```python
from build123d import *

# Parameters (mm, degrees)
SKETCH1_R           = 2.25
BOSS_EXTRUDE1_DEPTH = 3.5


with BuildPart() as part:
    # Sketch1 → Boss-Extrude1 (new body)
    with BuildSketch(Plane.XY):
        with BuildLine():
            Line((-100, 100), (-100, -100))
            Line((-100, -100), (-60.466933112, -100))
            ThreePointArc((-60.466933112, -100), (-38.490639688, 54.111358665), (92.5, -30))
            ThreePointArc((92.5, -30), (84.111358665, -68.490639688), (60.466933112, -100))
            Line((60.466933112, -100), (100, -100))
            Line((100, -100), (100, 32))
            Line((100, 32), (32, 100))
            Line((32, 100), (-100, 100))
        make_face()
        with Locations((-96.15, -96.15)):
            Circle(SKETCH1_R, mode=Mode.SUBTRACT)
        with Locations((96.15, -96.15)):
            Circle(SKETCH1_R, mode=Mode.SUBTRACT)
        with Locations((-96.15, 96.15)):
            Circle(SKETCH1_R, mode=Mode.SUBTRACT)
    extrude(amount=BOSS_EXTRUDE1_DEPTH)


solid = part.part
```
Design review of the part built by this model. Coordinates are the model's own, in mm. Coordinates: 2 decimals unless noted, no trailing zeros. Order: outer loops, then holes, each group sorted by start corner. A loop starts at its lowest first (then second) coordinate and runs counter-clockwise, first axis right, second up. Notation, with made-up numbers: M 4.25,67 L 31.25,67 A18 cw 31.25,71 Z; hole C 63.25,24.25 d9. An arc over 180 degrees is marked long. Answer as a JSON object with one key per item and string values. Group by question number.
1) Add section A-A, the plane y = 60. Write out the cut boundary in (x, z).
2) Mouldability with a two-part tool opening along X and no side actions: class faces 1 (the cylindrical face through (-94.07, -97.01, 1.73)), 2 (the flat face through (-38, 60, 3.5)), 3 (the flat face through (66, 66, 2)) as pulls with the +X half, pulls with the -X half, needs draft (parallel to the pull), parting line crosses it, or undercut.
3) Add section D-D, the plane x = 36. Write out the cut boundary in (y, z), then the cut area to 3 significant figures.
4) Add section B-B, the plane z = 2.85. Write out the cut boundary in (x, y), then the cut area to 3 significant figures.
5) Add section C-C, the plane x = -69. Write out the cut boundary in (y, z), then the cut area to 3 significant figures.
6) Wall thickness on L1, parallel to Y at x = -96.15, z = 2.6; L2, parallel to X at y = -14, z = 3.1; L3, parallel to Y at x = -69.5, z = 0.85: over which ranges is each line inside the solid? List them lowest first.
Computed values:
{
 "1": {"outline": "M -100,0 L -21.36,0 L -21.36,3.5 L -100,3.5 Z; M 21.36,0 L 72,0 L 72,3.5 L 21.36,3.5 Z"},
 "2": {"face 1": "undercut", "face 2": "needs draft", "face 3": "pulls with the +X half"},
 "3": {"outline": "M 55.21,0 L 96,0 L 96,3.5 L 55.21,3.5 Z", "area": "143 mm^2"},
 "4": {"outline": "M -100,-100 L -60.47,-100 A92.5 cw long 60.47,-100 L 100,-100 L 100,32 L 32,100 L -100,100 Z; hole C -96.15,-96.15 d4.5; hole C -96.15,96.15 d4.5; hole C 96.15,-96.15 d4.5", "area": "12,600 mm^2"},
 "5": {"outline": "M -100,0 L -91.61,0 L -91.61,3.5 L -100,3.5 Z; M 31.61,0 L 100,0 L 100,3.5 L 31.61,3.5 Z", "area": "269 mm^2"},
 "6": {"L1": "y = -100 to -98.4, -93.9 to 93.9, 98.4 to 100", "L2": "x = -100 to -91.11, 91.11 to 100", "L3": "y = -100 to -91.04, 31.04 to 100"}
}
